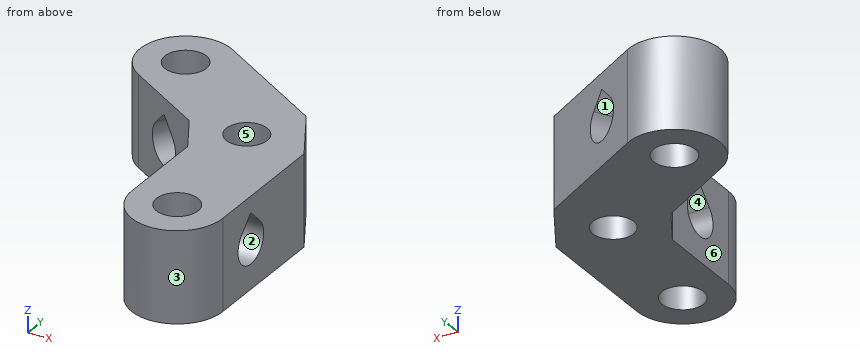
from build123d import *

# Parameters (mm, degrees)
BOSS_EXTRUDE1_DEPTH = 14
HOLE1_D             = 6.4
HOLE1_DEPTH         = 14
HOLE2_D             = 6.4
HOLE2_DEPTH         = 14
CUT_EXTRUDE1_DEPTH  = 27.088457268
CUT_EXTRUDE2_DEPTH  = 15
SKETCH8_R           = 3.15
CUT_EXTRUDE3_DEPTH  = 15


with BuildPart() as part:
    # Sketch1 → Boss-Extrude1 (new body)
    with BuildSketch(Plane.XY.offset(14)):
        with BuildLine():
            Line((7, 0), (7, 20.267949192))
            Line((7, 20.267949192), (2, 28.92820323))
            Line((2, 28.92820323), (-15.552558883, 39.062177826))
            ThreePointArc((-15.552558883, 39.062177826), (-25.11473671, 36.5), (-22.552558883, 26.937822174))
            Line((-22.552558883, 26.937822174), (-10.464101615, 19.958548116))
            Line((-10.464101615, 19.958548116), (-7, 13.958548116))
            Line((-7, 13.958548116), (-7, 0))
            ThreePointArc((-7, 0), (0, -7), (7, 0))
        make_face()
    extrude(amount=-BOSS_EXTRUDE1_DEPTH)

    # Hole1
    with Locations(Plane(origin=(0, 0, 0), x_dir=(-1, 0, 0), z_dir=(0, 0, -1))):
        with Locations((0, 0)):
            Hole(HOLE1_D / 2, depth=HOLE1_DEPTH)

    # Hole2
    with Locations(Plane(origin=(0, 0, 0), x_dir=(-1, 0, 0), z_dir=(0, 0, -1))):
        with Locations((19.0525, 32.999898011)):
            Hole(HOLE2_D / 2, depth=HOLE2_DEPTH)

    # Sketch2 → Cut-Extrude1 (cut, through all)
    with BuildSketch(Plane(origin=(6.026279442, 10.437822174, 0), x_dir=(0.866025404, -0.5, 0), z_dir=(-0.5, -0.866025404, 0))):
        with BuildLine():
            Line((-25.999898011, 11.5254834), (-28.262639711, 9.2627417))
            ThreePointArc((-28.262639711, 9.2627417), (-25.999898011, 3.8), (-23.737156311, 9.2627417))
            Line((-23.737156311, 9.2627417), (-25.999898011, 11.5254834))
        make_face()
    extrude(amount=-CUT_EXTRUDE1_DEPTH, mode=Mode.SUBTRACT)

    # Sketch3 → Cut-Extrude2 (cut, through all)
    with BuildSketch(Plane.ZY.offset(7)):
        with BuildLine():
            Line((9.2627417, 4.7372583), (11.5254834, 7))
            Line((11.5254834, 7), (9.2627417, 9.2627417))
            ThreePointArc((9.2627417, 9.2627417), (3.8, 7), (9.2627417, 4.7372583))
        make_face()
    extrude(amount=-CUT_EXTRUDE2_DEPTH, mode=Mode.SUBTRACT)

    # Sketch8 → Cut-Extrude3 (cut, through all)
    with BuildSketch(Plane.XY.offset(14)):
        with Locations((-2.116025404, 20.778312164)):
            Circle(SKETCH8_R)
    extrude(amount=-CUT_EXTRUDE3_DEPTH, mode=Mode.SUBTRACT)


solid = part.part
Design review of the part built by this model. Coordinates are the model's own, in mm. Face numbers are marked on the shaded views. A direction names the side the tool comes from. Give positions to 0.01 mm unless a question says otherwise; leave off trailing zeros. Write each loop counter-clockwise with the first axis right and the second up, starting at its lowest first coordinate (ties: lowest second). Pieces come first, ordered by that corner, then holes. Notation, with made-up numbers: M 29,21.25 L 76,21.25 A20 cw 76,45.25 Z; hole C -37.75,-16.75 d11. An arc over 180 degrees is marked long. Return JSON: item names as keys, results as strings. Group by question number.
Item 1: Tool access review of the marked faces 4, 5 and 6: name each direction out of +Z, -Z, +X, -X, +Y, -Y from which nothing blocks a thin tool from reaching the whole face with its end or side.
Item 2: Take a section at D-D (z = 1.25). Give the boundary of the cut face in (x, y), plus the area to 3 significant figures.
Item 3: The part is to be moulded in two halves that separate along X. For the marked faces 1, 2 and 3, say which applies: pulls with the +X half, pulls with the -X half, needs draft (parallel to the pull), parting line crosses it, or undercut.
Item 4: Clearance check with flat-ended pins moving along their axes: pin 1 Ø6 at (x, y) = (0, 0) entering from -Z; pin 2 Ø3 at (x, z) = (-22, 6) entering from +Y; pin 3 Ø5 at (x, z) = (-13.5, 11.5) entering from -Y; pin 4 Ø7 at (y, z) = (4.5, 7) entering from -X. State where each tip first meets the part, or that it passes through.
Item 5: Take a section at A-A (z = 5.75). Count the separate pieces of the cut face and the enclosed holes in it, plus the area to 3 significant figures.
Item 6: Take a section at B-B (x = 0). Give the boundary of the cut face in (y, z), plus the area to 3 significant figures.
Item 7: Take a section at C-C (x = -21). Give the boundary of the cut face in (y, z).
Item 8: Wall thickness on line 1 along Y through (x, z) = (0, 11.25); line 2 along Y through (x, z) = (-13, 8.5); line 3 along Y through (x, z) = (-0.5, 9.5): over which ranges is each line inside the solid? List them lowest first.
Return value:
{
 "1": {"face 4": "+X, -X", "face 5": "+Z, -Z", "face 6": "+Z, -Z, -X, -Y"},
 "2": {"outline": "M -22.55,26.94 L -10.46,19.96 L -7,13.96 L -7,0 A7 ccw 7,0 L 7,20.27 L 2,28.93 L -15.55,39.06 A7 ccw Z; hole C -19.05,33 d6.4; hole C -2.12,20.78 d6.3; hole C 0,0 d6.4", "area": "667 mm2"},
 "3": {"face 1": "undercut", "face 2": "needs draft", "face 3": "parting line crosses it"},
 "4": {"pin 1": "passes through", "pin 2": "stops at y = 39.85", "pin 3": "stops at y = 20.27", "pin 4": "stops at x = -7"},
 "5": {"separate pieces": "3", "enclosed holes": "3", "area": "502 mm2"},
 "6": {"outline": "M -7,0 L -3.2,0 L -3.2,14 L -7,14 Z; M 3.2,0 L 18.44,0 L 18.44,14 L 3.2,14 Z; M 23.11,0 L 30.08,0 L 30.08,14 L 23.11,14 Z; hole M 4.74,9.26 A3.2 ccw long 9.26,9.26 L 7,11.53 Z", "area": "330 mm2"},
 "7": {"outline": "M 26.04,0 L 30.46,0 L 30.46,14 L 26.04,14 Z; M 35.54,0 L 39.72,0 L 39.72,14 L 35.54,14 Z"},
 "8": {"line 1": "y = -7 to -3.2, 3.2 to 6.72, 7.28 to 18.44, 23.11 to 30.08", "line 2": "y = 21.42 to 23.83, 35.14 to 37.59", "line 3": "y = -6.98 to -3.16, 3.16 to 4.97, 9.03 to 18.07, 23.48 to 30.37"}
}
